For this review, take the finished solid that the model builds, in its own axes (mm). A direction names the side the tool comes from. Coordinates: 2 decimals unless noted, no trailing zeros. Write each loop counter-clockwise with the first axis right and the second up, starting at its lowest first coordinate (ties: lowest second). Pieces come first, ordered by that corner, then holes. Notation, with made-up numbers: M 43.25,63.5 L 50.25,63.5 A16 ccw 50.25,92.5 Z; hole C 40,2 d7. An arc over 180 degrees is marked long. One line per question, with ' | ' between items.
Autodesk Inventor part; units mm, degrees
ref_plane "YZ Plane" through (0, 0, 0) normal (1, 0, 0) x (0, 1, 0)
ref_plane "XZ Plane" through (0, 0, 0) normal (0, 1, 0) x (-1, 0, 0)
ref_plane "XY Plane" through (0, 0, 0) normal (0, 0, 1) x (1, 0, 0)
sketch "Sketch1" plane through (0, 0, 0) normal (0, 1, 0) x (-1, 0, 0)
  line L0 (17.5, 15) -> (-17.5, 15)
  line L1 (-17.5, 15) -> (-17.5, -15)
  line L2 (-17.5, -15) -> (17.5, -15)
  line L3 (17.5, -15) -> (17.5, 15)
  line L4 (17.5, 15) -> (-17.5, -15) construction
  line L5 (-17.5, 15) -> (17.5, -15) construction
  point P0 (0, 0)
  dimension "d0" = 35
  dimension "d1" = 30
extrude "Extrusion1" add sketch "Sketch1" along normal blind 1
sketch "Sketch2" plane through (0, 1, 0) normal (0, 1, 0) x (1, 0, 0)
  line L0 (-17.5, 15) -> (-17.5, -15)
  line L1 (-17.5, 0) -> (17.5, 0)
  line L2 (17.5, -15) -> (17.5, 15)
  line L3 (-17.5, -15) -> (17.5, -15)
  line L4 (0, -15) -> (0, 15)
  line L5 (17.5, 15) -> (-17.5, 15)
  point P0 (0, 0)
  point P1 (-15.025, -12.1525)
  point P2 (-15.025, 12.1525)
  point P3 (15.025, -12.1525)
  point P4 (15.025, 12.1525)
  dimension "d11" = 15.025
  dimension "d12" = 12.1525
hole "Hole1" at (-15.025, 1, 12.1525) at (-15.025, 1, -12.1525) at (15.025, 1, -12.1525) at (15.025, 1, 12.1525) direction (0, -1, 0) diameter 3.2 end through all
sketch "Sketch3" plane through (0, 1, 0) normal (0, 1, 0) x (1, 0, 0)
  circle A0 centre (0, 0) radius 13.5
  dimension "d13" = 27
extrude "Extrusion2" add sketch "Sketch3" along normal blind 3
sketch "Sketch4" plane through (0, 4, 0) normal (0, 1, 0) x (1, 0, 0)
  circle A0 centre (0, 0) radius 13.5
  line L0 (17.5, 15) -> (-17.5, 15)
  line L1 (-9.5, 15) -> (9.5, 15)
  line L2 (9.5, 15) -> (9.5, 8)
  line L3 (9.5, 8) -> (-9.5, 8)
  line L4 (-9.5, 8) -> (-9.5, 15)
  line L5 (-9.5, 15) -> (9.5, 8) construction
  line L6 (9.5, 15) -> (-9.5, 8) construction
  point P0 (0, 11.5)
  point P1 (0, 8)
  point P2 (-9.5, 9.5917)
  point P3 (9.5, 9.5917)
  dimension "d16" = 19
  dimension "d17" = 7
extrude "Extrusion3" add sketch "Sketch4" along normal blind 1
sketch "Sketch5" plane through (9.5, 4, -9.5917) normal (1, 0, 0) x (0, 0, -1)
  line L0 (0, 0) -> (5.4083, 0)
  line L1 (5.4083, 0) -> (11.637, 14.1369)
  arc A0 (11.637, 14.1369) -> (2.8827, 16.9336) centre (7.4083, 16) ccw
  line L2 (2.8827, 16.9336) -> (0, 0)
  line L3 (2.8827, 16.9336) -> (-18.8286, 1)
  line L4 (0, 1) -> (-23.0917, 1)
  line L5 (0, 1) -> (1.0062, 1)
  line L6 (5.4083, 1) -> (0, 1)
  point P0 (-9.5917, -4)
  point P1 (0.1702, 1)
  dimension "d20" = 16
  dimension "d31" = 2
extrude "Extrusion4" add sketch "Sketch5" against normal blind 1
mirror "Mirror1" about plane through (0, 0, 0) normal (1, 0, 0) of "Extrusion4"
fillet "Fillet2" radius 2 2 edges at (-9.5, 4.5, -9.5917) (9.5, 4.5, -9.5917)
sketch "Sketch6" plane through (0, 0, 0) normal (1, 0, 0) x (0, 1, 0)
  arc A0 (18.1369, -21.2287) -> (20.9336, -12.4744) centre (20, -17) ccw
  circle A1 centre (20, -17) radius 11.5
  point P0 (0, 0)
  dimension "d25" = 23
extrude "Extrusion5" add sketch "Sketch6" along normal mid plane 12
sketch "Sketch7" plane through (8.5, 4, -9.5917) normal (-1, 0, 0) x (0, 0, 1)
  arc A0 (-2.8827, 16.9336) -> (-11.637, 14.1369) centre (-7.4083, 16) ccw
  circle A1 centre (-7.4083, 16) radius 2.3211
  point P0 (9.5917, -4)
extrude "Extrusion6" add sketch "Sketch7" along normal up to surface (17 mm away)
fillet "Fillet3" radius 2 2 edges at (6, 8.5, -17) (-6, 8.5, -17)
properties part number "rearaxle" material "Stainless Steel AISI 440C, Welded"
1. Clearance check with flat-ended pins moving along their axes: P1, Ø5.5, axis at y = 17.5, z = -13.5, coming from the +X side; P2, Ø1.1, axis at x = 1.5, y = 0.5, coming from the -Z side; P3, Ø3.5, axis at x = -15.02, z = -12.15, coming from the +Y side; P4, Ø1.9, axis at x = -15.02, z = 12.15, coming from the -Y side. State where each tip first meets the part, or that it passes through.
Computed values:
P1: stops at x = 9.5 | P2: stops at z = -15 | P3: stops at y = 1 | P4: passes through
2. Draft analysis for pull direction Z (two halves, no side actions). For faces 1 (the flat face through (6, 22, -19)), 2 (the cylindrical face through (13.44, 0.49, -12.36)), 3 (the cylindrical face through (12.5, 3, 5.1)), state which applies: pulls with the +Z half, pulls with the -Z half, needs draft (parallel to the pull), parting line crosses it, or undercut.
Computed values:
face 1: needs draft | face 2: undercut | face 3: parting line crosses it
3. Take a section at D-D on y = 14.5. Give the number of separate pieces and of enclosed holes in the cut face, plus the area to 3 significant figures.
Computed values:
separate pieces: 3 | enclosed holes: 0 | area: 270 mm2
4. Take a section at C-C on y = 20. State the section outline as (x, z) points, plus the area to 3 significant figures.
Computed values:
outline: M -9.5,-21.62 L -8.5,-21.62 L -8.5,-19.32 L -6,-19.32 L -6,-26.5 A2 ccw -4,-28.5 L 4,-28.5 A2 ccw 6,-26.5 L 6,-19.32 L 8.5,-19.32 L 8.5,-21.62 L 9.5,-21.62 L 9.5,-11.2 L 8.5,-11.2 L 8.5,-14.68 L 6,-14.68 L 6,-7.5 A2 ccw 4,-5.5 L -4,-5.5 A2 ccw -6,-7.5 L -6,-14.68 L -8.5,-14.68 L -8.5,-11.2 L -9.5,-11.2 Z | area: 317 mm2
5. For line 1 along X through (y, z) = (9, -4.5); line 2 along Y through (x, z) = (7, -13.5); line 3 along Y through (x, z) = (11, 0), list the stretches that pass through material, from the lowest coordinate up.
Computed values:
line 1: x = -9.5 to -8.5, 8.5 to 9.5 | line 2: y = 0 to 1, 4 to 5 | line 3: y = 0 to 5
6. Machinability: for faces 4 (the flat face through (9.01, 10.97, -18.07)), 5 (the flat face through (9, 13.1, -1.8)), 6 (the flat face through (0.2, 0.5, -15)), which of the approach directions +Z, -Z, +X, -X, +Y, -Y give a long, thin tool a straight path to every point of the face, cutting with its end or side? Answer none if there is none.
Computed values:
face 4: -Z, +X, -Y | face 5: +Z, +X, +Y | face 6: -Z, +X, -X, -Y
7. Take a section at B-B on z = -17. State the section outline as (x, y) points, plus the area to 3 significant figures.
Computed values:
outline: M -9.5,8.54 L -8.5,8.54 L -8.5,17.68 L -6,17.68 L -6,10.5 A2 ccw -4,8.5 L 4,8.5 A2 ccw 6,10.5 L 6,17.68 L 8.5,17.68 L 8.5,8.54 L 9.5,8.54 L 9.5,24.62 L 8.5,24.62 L 8.5,22.32 L 6,22.32 L 6,29.5 A2 ccw 4,31.5 L -4,31.5 A2 ccw -6,29.5 L -6,22.32 L -8.5,22.32 L -8.5,24.62 L -9.5,24.62 Z | area: 328 mm2
8. Take a section at A-A on x = 0. State the section outline as (y, z) points, plus the area to 3 significant figures.
Computed values:
outline: M 0,-15 L 1,-15 L 1,-13.5 L 4,-13.5 L 4,-15 L 5,-15 L 5,13.5 L 1,13.5 L 1,15 L 0,15 Z; C 20,-17 d23 | area: 555 mm2
